The listing builds one solid part. Answer for the finished solid, in the listing's coordinates (mm). A direction names the side the tool comes from. Give positions to 0.01 mm unless a question says otherwise; leave off trailing zeros. Order: outer loops, then holes, each group sorted by start corner. A loop starts at its lowest first (then second) coordinate and runs counter-clockwise, first axis right, second up. Notation, with made-up numbers: (37.25, 59) - (92.25, 59) arc R20 cw to (92.25, 87) - close; hole circle Ø7 at (51.25, 23). An arc over 180 degrees is marked (long way). Use CSV: the item, a comma, the result in double quotes.
```python
from build123d import *

# Parameters (mm, degrees)
SKETCH_1_R               = 17
SKETCH_1_R_2             = 14
EXTRUDE_1_DEPTH          = 40
SKETCH_2_W               = 3
SKETCH_2_H               = 2
EXTRUDE_2_DEPTH          = 6
PATTERN_CIRCULAR_1_COUNT = 16


with BuildPart() as part:
    # 草图1 → 凸台-拉伸1 (new body)
    with BuildSketch(Plane(origin=(0, 0, 0), x_dir=(1, 0, 0), z_dir=(0, 1, 0))):
        Circle(SKETCH_1_R)
        Circle(SKETCH_1_R_2, mode=Mode.SUBTRACT)
    extrude(amount=EXTRUDE_1_DEPTH)

    # 草图2 → 凸台-拉伸2 (add)
    with BuildSketch(Plane(origin=(0, 0, 0), x_dir=(-1, 0, 0), z_dir=(0, -1, 0))):
        with Locations((0, 17)):
            Rectangle(SKETCH_2_W, SKETCH_2_H)
    extrude_2 = extrude(amount=-EXTRUDE_2_DEPTH)

    # 阵列(圆周)1: 凸台-拉伸2 ×16 about axis
    pattern_circular_1_axis = Axis((0, 0, 0), (0, 1, 0))
    for i in range(1, PATTERN_CIRCULAR_1_COUNT):
        add(extrude_2.rotate(pattern_circular_1_axis, i * 360 / PATTERN_CIRCULAR_1_COUNT))


solid = part.part
```
Item 1: Which of the six approach directions +Z, -Z, +X, -X, +Y, -Y give full straight-line access (tool end or side, diameter ignored) to faces 1 (the face through (-7, 6, -16)), 2 (the face through (5.296, 2.958, -16.704)), 3 (the face through (17.5, 3, 1.5)), 4 (the face through (12.4, 6, -12.3))?
Taken from the geometry:
face 1,"-Z, -X, +Y"
face 2,"-Z, +Y, -Y"
face 3,"+X, +Y, -Y"
face 4,"-Z, +X, +Y"
Item 2: The part is cut by section A-A (x = 0). Give the vertices of the cut face in (y, z), and give its area (3 significant figures).
Taken from the geometry:
outline,"(0, -18) - (6, -18) - (6, -17) - (40, -17) - (40, -14) - (0, -14) - close; (0, 14) - (40, 14) - (40, 17) - (6, 17) - (6, 18) - (0, 18) - close"
area,"252 mm^2"
Item 3: The mould has two halves that part along Z. Classify faces 5 (the face through (15.56, 2.96, 8.07)), 6 (the face through (-17.5, 3, 1.5)), 7 (the face through (-16.704, 2.958, -5.296)), 8 (the face through (18, 3, 0)): +Z half, -Z half, draft (parallel to the pull), parting line (faces both ways), or undercut.
Taken from the geometry:
face 5,"+Z half"
face 6,"undercut"
face 7,"undercut"
face 8,"draft"
Item 4: The part is cut by section C-C (y = 17.5). Give the vertices of the cut face in (x, z), and give its area (3 significant figures).
Taken from the geometry:
outline,"circle Ø34 at (0, 0); hole circle Ø28 at (0, 0)"
area,"292 mm^2"
Item 5: Each of these flat-tipped pins is pushed along its axis until it touches: pin 1 (0.9 mm diameter, centred on x = -17.5, y = 3, fed in from +Z); pin 2 (1.7 mm diameter, centred on x = -6.5, z = -16, fed in from +Y); pin 3 (4 mm diameter, centred on x = -4, y = 9.5, fed in from +Z); pin 4 (1 mm diameter, centred on y = 8, z = 8.5, fed in from -X). Where does it stop, or does it pass through?
Taken from the geometry:
pin 1,"z = 5.87"
pin 2,"y = 40"
pin 3,"z = 16.88"
pin 4,"x = -15"
Item 6: The part is cut by section B-B (z = 0). Give the vertices of the cut face in (x, y), and give its area (3 significant figures).
Taken from the geometry:
outline,"(-18, 0) - (-14, 0) - (-14, 40) - (-17, 40) - (-17, 6) - (-18, 6) - close; (14, 0) - (18, 0) - (18, 6) - (17, 6) - (17, 40) - (14, 40) - close"
area,"252 mm^2"
Item 7: Find the intervals of material crossed by line 1 along Z through (x, y) = (0, 13.5); line 2 along Z through (x, y) = (9, 21.5), in increasing order.
Taken from the geometry:
line 1,"-17 to -14, 14 to 17"
line 2,"-14.42 to -10.72, 10.72 to 14.42"
